from build123d import *

# Parameters (mm, degrees)
F0_W     = 26
F0_H     = 2
F1_DEPTH = 30
F0_H_2   = 34
F2_DEPTH = 2
F4_DEPTH = 28
F5_R     = 5
F6_R     = 5
F9_DEPTH = 100


# Not quite as in the source:
# - a feature of the source that left no trace in its solid (it failed there, or was rolled back) is left out


with BuildPart() as f1:
    # F0 (on Top) → F1 (new body)
    with BuildSketch(Plane.XY):
        with Locations((0, 17)):
            Rectangle(F0_W, F0_H)
    extrude(amount=F1_DEPTH)

    # F0 (on Top) → F2 (join)
    with BuildSketch(Plane.XY):
        with Locations((0, -1)):
            Rectangle(F0_W, F0_H_2)
    extrude(amount=F2_DEPTH)

    # F3 (on face) → F4 (join)
    with BuildSketch(Plane.XY.offset(2)):
        Polygon((13, -16), (0, -16), (-13, -16), (-13, -18), (13, -18), align=None)
    extrude(amount=F4_DEPTH)

    # F5
    f5_edges = [f1.edges().sort_by_distance(p)[0] for p in [
        (-13, 17, 30),
        (-13, -17, 30),
    ]]
    fillet(f5_edges, radius=F5_R)

    # F6
    f6_edges = [f1.edges().sort_by_distance(p)[0] for p in [
        (13, 17, 30),
        (13, -17, 30),
    ]]
    fillet(f6_edges, radius=F6_R)

    # F8 (on face) → F9 (cut)
    with BuildSketch(Plane(origin=(0, 18, 0), x_dir=(-1, 0, 0), z_dir=(0, 1, 0))):
        with BuildLine():
            ThreePointArc((5, 15), (3.5355339059, 18.5355339059), (0, 20))
            Line((0, 20), (0, 10))
            ThreePointArc((0, 10), (3.5355339059, 11.4644660941), (5, 15))
        make_face()
        with BuildLine():
            Line((0, 10), (0, 20))
            ThreePointArc((0, 20), (-5, 15), (0, 10))
        make_face()
    extrude(amount=-F9_DEPTH, mode=Mode.SUBTRACT)


solid = f1.part
Verification items for the finished model (mm, model axes). A direction names the side the tool comes from. Coordinates: 2 decimals unless noted, no trailing zeros. Write each loop counter-clockwise with the first axis right and the second up, starting at its lowest first coordinate (ties: lowest second). Pieces come first, ordered by that corner, then holes. Notation, with made-up numbers: M 17.5,62 L 61.5,62 A35 ccw 61.5,98 Z; hole C 71.25,61 d8. An arc over 180 degrees is marked long. Use a Markdown table: item, result.
Q1. Go/stop test with a flat-tipped pin: P1, Ø12, axis at x = -2.5, y = 5, coming from the +Z side. Record where the tip stops, or that it passes through.
Reply:
| item | result |
|---|---|
| P1 | stops at z = 2 |
Q2. Sectioned sample at A-A, the plane z = 13. Record the boundary of the cut face in (x, y), plus the area to 3 significant figures.
Reply:
| item | result |
|---|---|
| outline | M -13,-18 L -4.58,-18 L -4.58,-16 L -13,-16 Z; M -13,16 L -4.58,16 L -4.58,18 L -13,18 Z; M 4.58,-18 L 13,-18 L 13,-16 L 4.58,-16 Z; M 4.58,16 L 13,16 L 13,18 L 4.58,18 Z |
| area | 67.3 mm² |
Q3. Thickness scan on line 1 (Y direction, x = -8.5, z = 24); line 2 (Z direction, x = 8, y = 15). Record the ranges inside material, lowest first.
Reply:
| item | result |
|---|---|
| line 1 | y = -18 to -16, 16 to 18 |
| line 2 | z = 0 to 2 |
Q4. Set-up check for faces 4 (the face through (-6, 16, 16)), 5 (the face through (13, -4, 1)): record each of +Z, -Z, +X, -X, +Y, -Y from which the full face is reachable in a straight line by a thin tool's end or side.
Reply:
| item | result |
|---|---|
| face 4 | +Z, +X, -X |
| face 5 | +Z, -Z, +X, +Y, -Y |
Q5. Draft check along Y on faces 1 (the face through (0, 0, 2)), 2 (the face through (-11, 17, 29)), 3 (the face through (-6, -18, 15)). Enter one of: +Y half, -Y half, draft (parallel to the pull), parting line (faces both ways), or undercut.
Reply:
| item | result |
|---|---|
| face 1 | undercut |
| face 2 | draft |
| face 3 | -Y half |
Q6. Sectioned sample at D-D, the plane x = 2.75. Record the boundary of the cut face in (y, z), plus the area to 3 significant figures.
Reply:
| item | result |
|---|---|
| outline | M -18,0 L 18,0 L 18,10.82 L 16,10.82 L 16,2 L -16,2 L -16,10.82 L -18,10.82 Z; M -18,19.18 L -16,19.18 L -16,30 L -18,30 Z; M 16,19.18 L 18,19.18 L 18,30 L 16,30 Z |
| area | 151 mm² |
Q7. Sectioned sample at B-B, the plane x = 5.75. Record the boundary of the cut face in (y, z).
Reply:
| item | result |
|---|---|
| outline | M -18,0 L 18,0 L 18,30 L 16,30 L 16,2 L -16,2 L -16,30 L -18,30 Z |
Q8. Sectioned sample at C-C, the plane z = 6. Record the boundary of the cut face in (x, y), plus the area to 3 significant figures.
Reply:
| item | result |
|---|---|
| outline | M -13,-18 L 13,-18 L 13,-16 L -13,-16 Z; M -13,16 L 13,16 L 13,18 L -13,18 Z |
| area | 104 mm² |
